Source: CAD feature listing. Evaluate the final solid. Frame: model axes, mm. Face numbers are marked on the shaded views. Round coordinates to 2 decimals unless told otherwise and drop trailing zeros. Write each loop counter-clockwise with the first axis right and the second up, starting at its lowest first coordinate (ties: lowest second). Pieces come first, ordered by that corner, then holes. Notation, with made-up numbers: (46, 73.25) - (70, 73.25) arc R37 ccw to (70, 112.25) - close; hole circle Ø10 at (-20, 42). An arc over 180 degrees is marked (long way). Write item = value, one per line. Start each with the question number.
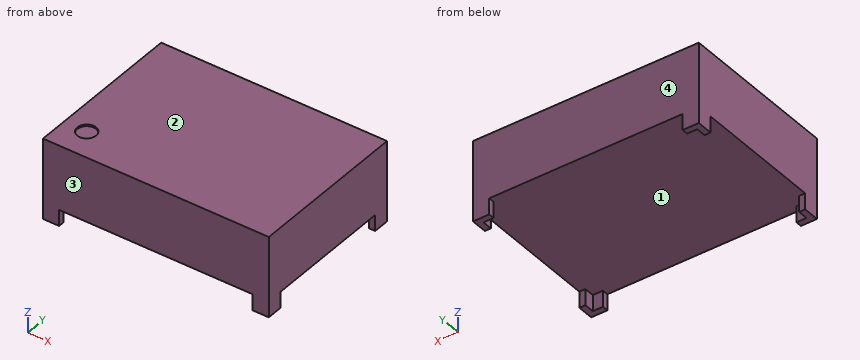
```python
from build123d import *

# Parameters (mm, degrees)
SKETCH_1_W          = 28
SKETCH_1_H          = 20
EXTRUDE_1_DEPTH     = 8
EXTRUDE_2_DEPTH     = 2
SKETCH_3_R          = 1.170120389
CUT_EXTRUDE_1_DEPTH = 0.2


with BuildPart() as part:
    # 草图1 → 拉伸1 (new body)
    with BuildSketch(Plane.XY):
        Rectangle(SKETCH_1_W, SKETCH_1_H)
    extrude(amount=EXTRUDE_1_DEPTH)

    # 草图2 → 拉伸2 (add)
    with BuildSketch(Plane(origin=(0, 0, 0), x_dir=(-1, 0, 0), z_dir=(0, 0, -1))):
        Polygon((-14, 10), (-14, 8), (-13.25, 8), (-13.25, 9.25), (-12, 9.25), (-12, 10), align=None)
        Polygon((12, 10), (14, 10), (14, 8), (13.25, 8), (13.25, 9.25), (12, 9.25), align=None)
        Polygon((-12, -10), (-14, -10), (-14, -8), (-13.25, -8), (-13.25, -9.25), (-12, -9.25), align=None)
        Polygon((14, -10), (14, -8), (13.25, -8), (13.25, -9.25), (12, -9.25), (12, -10), align=None)
    extrude(amount=EXTRUDE_2_DEPTH)

    # 草图3 → 切除-拉伸1 (cut)
    with BuildSketch(Plane.XY.offset(8)):
        with Locations((-11.177269576, -6.453473504)):
            Circle(SKETCH_3_R)
    extrude(amount=-CUT_EXTRUDE_1_DEPTH, mode=Mode.SUBTRACT)


solid = part.part
```
(1) Section A-A (x = -6.5). Return the cut outline in (y, z), plus the area to 3 significant figures.
(2) Contact query for flat-ended pins moving along their axis: P1, Ø12, axis at x = -1, y = 2.5, coming from the -Z side; P2, Ø2, axis at x = -11.18, y = -6.45, coming from the +Z side. Output: stop coordinate, or through.
(3) Section C-C (y = -7). Return the cut outline in (x, z), plus the area to 3 significant figures.
(4) Pull-direction query (Y, two-part tool) for the marked faces 1, 2, 3 and 4; classes: +Y half, -Y half, draft (parallel to the pull), parting line (faces both ways), or undercut.
(5) Ray query, L1, parallel to Z at x = -4.75, y = 1. Return the intervals inside material, ascending. Write a range as from..to.
(6) Section B-B (y = 6.5). Return the cut outline in (x, z), plus the area to 3 significant figures.
Solution:
q1.outline = (-10, 0) - (10, 0) - (10, 8) - (-10, 8) - close
q1.area = 160 mm^2
q2.P1 = 0
q2.P2 = 7.8
q3.outline = (-14, 0) - (14, 0) - (14, 8) - (-10.14, 8) - (-10.14, 7.8) - (-12.21, 7.8) - (-12.21, 8) - (-14, 8) - close
q3.area = 224 mm^2
q4.face_1 = undercut
q4.face_2 = draft
q4.face_3 = -Y half
q4.face_4 = +Y half
q5.L1 = 0..8
q6.outline = (-14, 0) - (14, 0) - (14, 8) - (-14, 8) - close
q6.area = 224 mm^2
